Part model, mm, in its own coordinate system. A direction names the side the tool comes from. Coordinates: 2 decimals unless noted, no trailing zeros. Loops run counter-clockwise (first coordinate to the right, second up) from the corner with the lowest first, then second, coordinate; pieces in that order, holes last. Notation, with made-up numbers: M 3,84 L 45,84 A8 cw 45,89 Z; hole C 72,84.5 d2. An arc over 180 degrees is marked long. Use a Markdown table: item, result. Add a question column.
1) Band-saw the part on B-B (y = 285.75). List the corners of the cut face in (x, z) (3 decimals), plus the area to 3 significant figures.
2) Tool access for faces 4 (the flat face through (7.95, 294, 51)), 5 (the cylindrical face through (97.78, 3.62, 51.51)): list every direction of +Z, -Z, +X, -X, +Y, -Y with a clear straight run to the whole face (end or side of a thin tool).
3) Pull direction Z, two halves, no side cores. Call faces 1 (the flat face through (50, 290, 101.6)), 2 (the cylindrical face through (3.93, 292.98, 41.36)), 3 (the flat face through (50, 290, 0)): released by +Z, released by -Z, zero draft, split by the parting line, or undercut.
4) Pin check, flat tip, straight feed: pin 1 Ø19 at (y, z) = (285.75, 50.8) entering from -X. Stop position of the tip, or through.
5) Wall check: probe 1 along Y at (x, z) = (42, 50); probe 2 along Z at (x, y) = (52.5, 285.75); probe 3 along Z at (x, y) = (2, 285.75). Give the ranges that are in metal, low to high. Write a range as from..to.
6) Band-saw the part on A-A (z = 50.8). List the corners of the cut face in (x, y) (3 decimals).
from build123d import *

# Parameters (mm, degrees)
SKETCH1_W           = 101.6
SKETCH1_H           = 558.8
BOSS_EXTRUDE1_DEPTH = 101.6
FILLET2_R           = 12.7


with BuildPart() as part:
    # Sketch1 → Boss-Extrude1 (new body)
    with BuildSketch(Plane.XY):
        with Locations((50.8, 279.4)):
            Rectangle(SKETCH1_W, SKETCH1_H)
    extrude(amount=BOSS_EXTRUDE1_DEPTH)

    # Fillet2
    fillet2_edges = [part.edges().sort_by_distance(p)[0] for p in [
        (50.8, 0, 0),
        (101.6, 0, 50.8),
        (0, 0, 50.8),
        (50.8, 0, 101.6),
    ]]
    fillet(fillet2_edges, radius=FILLET2_R)

    # Sketch8 → CBORE for M12 Hex Head Bolt1 (revolve, cut)
    with BuildSketch(Plane(origin=(0, 285.75, 50.8), x_dir=(0, 0, 1), z_dir=(0, 1, 0))):
        Polygon((0, 0), (0, 101.6), (7.5, 101.6), (7.5, 7.95), (11.89, 7.95), (11.89, 0.025), (11.915, 0), align=None)
    revolve(axis=Axis((-6.35, 285.75, 50.8), (1, 0, 0)), mode=Mode.SUBTRACT)


solid = part.part
Entries:
| question | item | result |
|---|---|---|
| 1 | outline | M 0,0 L 101.6,0 L 101.6,43.3 L 7.95,43.3 L 7.95,38.91 L 0.025,38.91 L 0,38.885 Z; M 0,62.715 L 0.025,62.69 L 7.95,62.69 L 7.95,58.3 L 101.6,58.3 L 101.6,101.6 L 0,101.6 Z |
| 1 | area | 8,730 mm2 |
| 2 | face 4 | -X |
| 2 | face 5 | +Z, -Z, +X, -Y |
| 3 | face 1 | released by +Z |
| 3 | face 2 | undercut |
| 3 | face 3 | released by -Z |
| 4 | pin 1 | x = 7.95 |
| 5 | probe 1 | 0..278.29, 293.21..558.8 |
| 5 | probe 2 | 0..43.3, 58.3..101.6 |
| 5 | probe 3 | 0..38.91, 62.69..101.6 |
| 6 | outline | M 0,12.7 A12.7 ccw 12.7,0 L 88.9,0 A12.7 ccw 101.6,12.7 L 101.6,278.25 L 7.95,278.25 L 7.95,273.86 L 0.025,273.86 L 0,273.835 Z; M 0,297.665 L 0.025,297.64 L 7.95,297.64 L 7.95,293.25 L 101.6,293.25 L 101.6,558.8 L 0,558.8 Z |
